from build123d import *

# Parameters (mm, degrees)
F1_DEPTH = 41
F3_DEPTH = 19
F4_R     = 5.402873
F5_DEPTH = 127


with BuildPart() as f1:
    # F0 (on Top) → F1 (new body)
    with BuildSketch(Plane.XY):
        Polygon((-42.681199, 31.584967), (-41.684866, -18.23815), (18.126922, -18.23815), (49.872324, 7.42222), (18.126922, 31.584967), align=None)
    extrude(amount=F1_DEPTH)

    # F2 (on face) → F3 (join)
    with BuildSketch(Plane.XY.offset(41)):
        Polygon((6.816162, 19.731937), (-29.038044, 19.731937), (-26.485959, 0), (8.835195, 0), align=None)
    extrude(amount=F3_DEPTH)

    # F4 (on face) → F5 (join)
    with BuildSketch(Plane(origin=(8.743648, 0.894677, 0), x_dir=(-0.101792, 0.994806, 0), z_dir=(0.994806, 0.101792, 0))):
        with Locations((9.018134, 51.709723)):
            Circle(F4_R)
    extrude(amount=F5_DEPTH)


solid = f1.part
Model file for the job. Use its own axes, mm. A direction names the side the tool comes from. Round coordinates to 2 decimals unless told otherwise and drop trailing zeros. Order: outer loops, then holes, each group sorted by start corner. A loop starts at its lowest first (then second) coordinate and runs counter-clockwise, first axis right, second up.
(1) Band-saw the part on C-C (y = 2.5). List the corners of the cut face in (x, z), then the cut area to 3 significant figures.
(2) Band-saw the part on A-A (x = 4.5). List the corners of the cut face in (y, z), then the cut area to 3 significant figures.
(3) Band-saw the part on B-B (z = 19.5). List the corners of the cut face in (x, y), then the cut area to 3 significant figures.
(4) Band-saw the part on D-D (y = -12). List the corners of the cut face in (x, z), then the cut area to 3 significant figures.
(5) 3-axis set-ups, long thin cutter, end or side, ignore diameter. For faces 4 (the face through (-9, 0, 50)), 5 (the face through (-11, 19.732, 50)), 6 (the face through (-27.78, 10, 50.37)), 7 (the face through (7.84, 9.73, 46.14)): which of +Z, -Z, +X, -X, +Y, -Y reach the whole face in a straight line?
(6) Drill centre lines: line 1 (Z direction, x = 7, y = -2); line 2 (X direction, y = 11.5, z = 17); line 3 (X direction, y = -3, z = 27). Where is each one in solid material? Low to high.
(7) Pin check, flat tips, straight feed: pin 1 (10 mm diameter, centred on y = 6, z = 19.5, fed in from +X); pin 2 (12 mm diameter, centred on y = 3.5, z = 52, fed in from -X); pin 3 (10 mm diameter, centred on y = 23, z = 46.5, fed in from +X). Stop position of each tip, or through.
(8) Pull direction Z, two halves, no side cores. Call faces 1 (the face through (-10, 10, 60)), 2 (the face through (134.174, 22.718, 51.785)), 3 (the face through (70.231, 15.074, 46.435)): released by +Z, released by -Z, zero draft, split by the parting line, or undercut.
Verdict:
1. outline: (-42.1, 0) - (43.78, 0) - (43.78, 41) - (8.58, 41) - (8.58, 60) - (-26.81, 60) - (-26.81, 41) - (-42.1, 41) - close
1. area: 4,190 mm2
2. outline: (-18.24, 0) - (31.58, 0) - (31.58, 41) - (19.73, 41) - (19.73, 60) - (0, 60) - (0, 41) - (-18.24, 41) - close
2. area: 2,420 mm2
3. outline: (-42.68, 31.58) - (-41.68, -18.24) - (18.13, -18.24) - (49.87, 7.42) - (18.13, 31.58) - close
3. area: 3,800 mm2
4. outline: (-41.81, 0) - (25.84, 0) - (25.84, 41) - (-41.81, 41) - close
4. area: 2,770 mm2
5. face 4: +Z, +X, -X, -Y
5. face 5: +Z, -X, +Y
5. face 6: +Z, -X, -Y
5. face 7: none
6. line 1: z = 0 to 41
6. line 2: x = -42.28 to 44.51
6. line 3: x = -41.99 to 36.98
7. pin 1: stops at x = 49.87
7. pin 2: stops at x = -27.71
7. pin 3: stops at x = 134.61
8. face 1: released by +Z
8. face 2: zero draft
8. face 3: undercut
